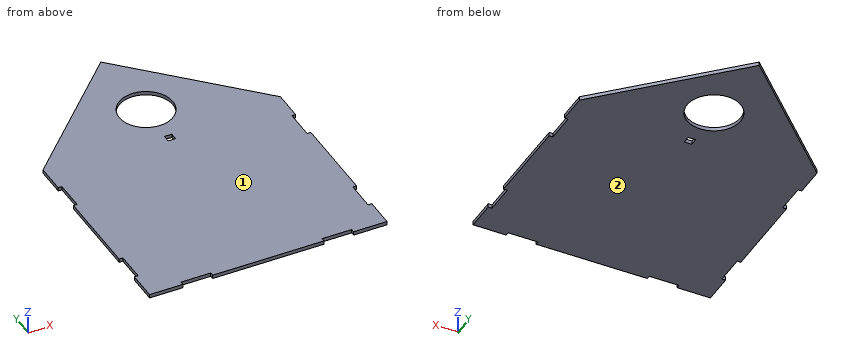
from build123d import *

# Parameters (mm, degrees)
BOSS_EXTRUDE1_DEPTH = 3.175
SKETCH3_R           = 22.86
CUT_EXTRUDE1_DEPTH  = 3.175
SKETCH5_W           = 6.35
SKETCH5_H           = 6.35
CUT_EXTRUDE2_DEPTH  = 3.175


with BuildPart() as part:
    # Sketch2 → Boss-Extrude1 (new body)
    with BuildSketch(Plane.XY):
        Polygon((0.564315933, 279.4), (-101.035684067, 177.8), (-101.035684067, 152.4), (-97.860684067, 152.4), (-97.860684067, 127), (-101.035684067, 127), (-101.035684067, 50.8), (-97.860684067, 50.8), (-97.860684067, 25.4), (-101.035684067, 25.4), (-101.035684067, 0), (-72.460684067, 0), (-72.460684067, 3.175), (-47.060684067, 3.175), (-47.060684067, 0), (48.189315933, 0), (48.189315933, 3.175), (73.589315933, 3.175), (73.589315933, 0), (102.164315933, 0), (102.164315933, 25.4), (98.989315933, 25.4), (98.989315933, 50.8), (102.164315933, 50.8), (102.164315933, 127), (98.989315933, 127), (98.989315933, 152.4), (102.164315933, 152.4), (102.164315933, 177.8), align=None)
    extrude(amount=BOSS_EXTRUDE1_DEPTH)

    # Sketch3 → Cut-Extrude1 (cut)
    with BuildSketch(Plane.XY.offset(3.175)):
        with Locations((3.739315933, 210.078311119)):
            Circle(SKETCH3_R)
    extrude(amount=-CUT_EXTRUDE1_DEPTH, mode=Mode.SUBTRACT)

    # Sketch5 → Cut-Extrude2 (cut)
    with BuildSketch(Plane.XY.offset(3.175)):
        with Locations((3.739315933, 170.159778504)):
            Rectangle(SKETCH5_W, SKETCH5_H)
    extrude(amount=-CUT_EXTRUDE2_DEPTH, mode=Mode.SUBTRACT)


solid = part.part
Build history of the part. All positions in model axes, mm. Face numbers are marked on the shaded views. Round coordinates to 2 decimals unless told otherwise and drop trailing zeros. Write each loop counter-clockwise with the first axis right and the second up, starting at its lowest first coordinate (ties: lowest second). Pieces come first, ordered by that corner, then holes. Notation, with made-up numbers: M -28.5,55 L 27.5,55 A21 cw 27.5,59 Z; hole C 27.5,8.5 d8. An arc over 180 degrees is marked long. Answer as a JSON object with one key per item and string values. Group by question number.
(1) Cut at B-B (x = -11). Give the cut face in (y, z) (3 decimals), and give its area (3 significant figures).
(2) Drill centre lines: L1, parallel to X at y = 136.5, z = 2.65; L2, parallel to X at y = 224, z = 1.65; L3, parallel to Y at x = -13, z = 2.7. Where is each one in solid material? Low to high.
(3) Cut at C-C (z = 1.2). Give the number of separate pieces and of enclosed holes in the cut face, and give its area (3 significant figures).
(4) Mould opens along Z. For the marked faces 1 and 2 say: pulls with the +Z half, pulls with the -Z half, needs draft (parallel to the pull), parting line crosses it, or undercut.
(5) Cut at A-A (y = 191.5). Give the cut face in (x, z) (3 decimals), and give its area (3 significant figures).
(6) Flat gauge pins, fed straight in: pin 1 (1 mm diameter, centred on y = 37, z = 1.5, fed in from -X); pin 2 (1 mm diameter, centred on y = 36, z = 1, fed in from +X); pin 3 (1.6 mm diameter, centred on x = -99.5, z = 2, fed in from -Y); pin 4 (1.6 mm diameter, centred on x = 57.5, z = 1.5, fed in from -Y) (3 decimals). Where does each tip first touch, or does it go through?
(7) Cut at D-D (y = 134.5). Give the cut face in (x, z) (3 decimals).
Responses:
{
 "1": {"outline": "M 0,0 L 192.605,0 L 192.605,3.175 L 0,3.175 Z; M 227.552,0 L 267.836,0 L 267.836,3.175 L 227.552,3.175 Z", "area": "739 mm2"},
 "2": {"L1": "x = -97.86 to 98.99", "L2": "x = -54.84 to -14.39, 21.87 to 55.96", "L3": "y = 0 to 194.51, 225.65 to 265.84"},
 "3": {"separate pieces": "1", "enclosed holes": "2", "area": "44,300 mm2"},
 "4": {"face 1": "pulls with the +Z half", "face 2": "pulls with the -Z half"},
 "5": {"outline": "M -87.336,0 L -9.581,0 L -9.581,3.175 L -87.336,3.175 Z; M 17.059,0 L 88.464,0 L 88.464,3.175 L 17.059,3.175 Z", "area": "474 mm2"},
 "6": {"pin 1": "stops at x = -97.86", "pin 2": "stops at x = 98.99", "pin 3": "stops at y = 0", "pin 4": "stops at y = 3.175"},
 "7": {"outline": "M -97.861,0 L 98.989,0 L 98.989,3.175 L -97.861,3.175 Z"}
}
